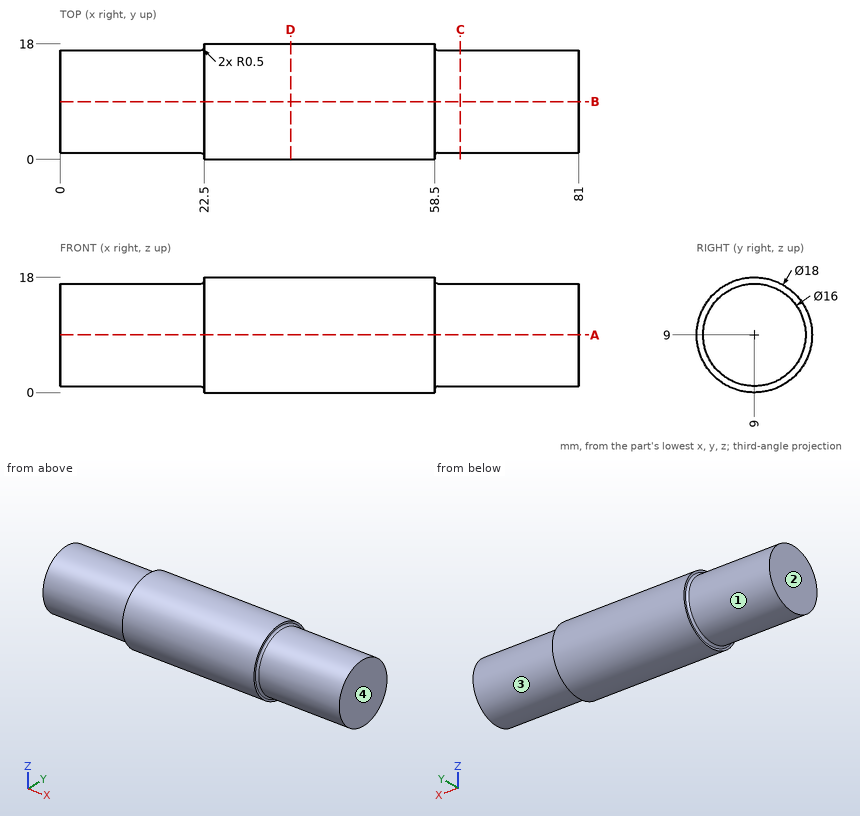
Input: dimensioned drawing with shaded views. Units: mm. Origin: part minimum x, y, z. A direction names the side the tool comes from. Coordinates: 2 decimals unless noted, no trailing zeros. Order: outer loops, then holes, each group sorted by start corner. A loop starts at its lowest first (then second) coordinate and runs counter-clockwise, first axis right, second up. Notation, with made-up numbers: M 44,-11.75 L 70,-11.75 A13 cw 70,13.25 Z; hole C 26.5,2 d5. An arc over 180 degrees is marked long. Answer as CSV lines item,"result".
Q1. Line query: probe 1 along X at (y, z) = (2.75, 15); probe 2 along Y at (x, z) = (11, 9.25); probe 3 along Y at (x, z) = (77.5, 11.5). Output: solid intervals per line, ascending. Write a range as [from, to].
Answers:
probe 1,"x = [22.5, 58.5]"
probe 2,"y = [1, 17]"
probe 3,"y = [1.4, 16.6]"
Q2. Section A-A on z = 9. Return the cut outline in (x, y), and give its area (3 significant figures).
Answers:
outline,"M 0,1 L 22,1 A0.5 cw 22.5,0.5 L 22.5,0 L 58.5,0 L 58.5,0.5 A0.5 cw 59,1 L 81,1 L 81,17 L 59,17 A0.5 cw 58.5,17.5 L 58.5,18 L 22.5,18 L 22.5,17.5 A0.5 cw 22,17 L 0,17 Z"
area,"1,370 mm^2"
Q3. Section C-C on x = 62.5. Return the cut outline in (y, z), and give its area (3 significant figures).
Answers:
outline,"C 9,9 d16"
area,"201 mm^2"
Q4. Set-up query: the marked faces 3 and 4. Return all of +Z, -Z, +X, -X, +Y, -Y with unobstructed straight access to the full face (end or side cutting, diameter ignored); none if empty.
Answers:
face 3,"+X"
face 4,"+Z, -Z, +X, +Y, -Y"
Q5. First-contact query: P1, Ø1, axis at x = 37.5, y = 6.5, coming from the +Z side; P2, Ø6, axis at x = 18, y = 12.5, coming from the -Z side; P3, Ø2, axis at x = 56, z = 15, coming from the -Y side. Flat tips, straight axial feed; report the tip coordinate or a pass-through.
Answers:
P1,"stops at z = 17.77"
P2,"stops at z = 1.02"
P3,"stops at y = 1.52"
Q6. Section D-D on x = 36. Return the cut outline in (y, z), and give its area (3 significant figures).
Answers:
outline,"C 9,9 d18"
area,"254 mm^2"
Q7. Draft query along Z for the marked faces 1 and 2. Return one class per face: pulls with the +Z half, pulls with the -Z half, needs draft (parallel to the pull), parting line crosses it, or undercut.
Answers:
face 1,"parting line crosses it"
face 2,"needs draft"
